Can you work these out from the drawing? Everything is in mm from the part's minimum corner. Coordinates: 2 decimals unless noted, no trailing zeros. Write each loop counter-clockwise with the first axis right and the second up, starting at its lowest first coordinate (ties: lowest second). Pieces come first, ordered by that corner, then holes.
(1) Imagine slicing it at C-C, the plane y = 450. List the corners of the cut face in (x, z) for me.
(2) For pin 1 Ø10 at (y, z) = (107.5, 7) entering from -X; pin 2 Ø12 at (y, z) = (646.5, 8.5) entering from -X, each with a flat end and sliding along its axis, tell me the tip position at first contact or that it passes through.
(3) Imagine slicing it at D-D, the plane y = 982. List the corners of the cut face in (x, z) for me.
(4) Imagine slicing it at A-A, the plane x = 766.5. List the corners of the cut face in (y, z) for me, plus the area to 3 significant figures.
(5) Imagine slicing it at B-B, the plane z = 14.5. List the corners of the cut face in (x, y) for me.
(6) Please list where these lines run through material, in increasing order: probe 1 along Y at (x, z) = (915, 17); probe 2 along X at (y, z) = (548, 7.75); probe 3 along X at (y, z) = (620, 4.5).
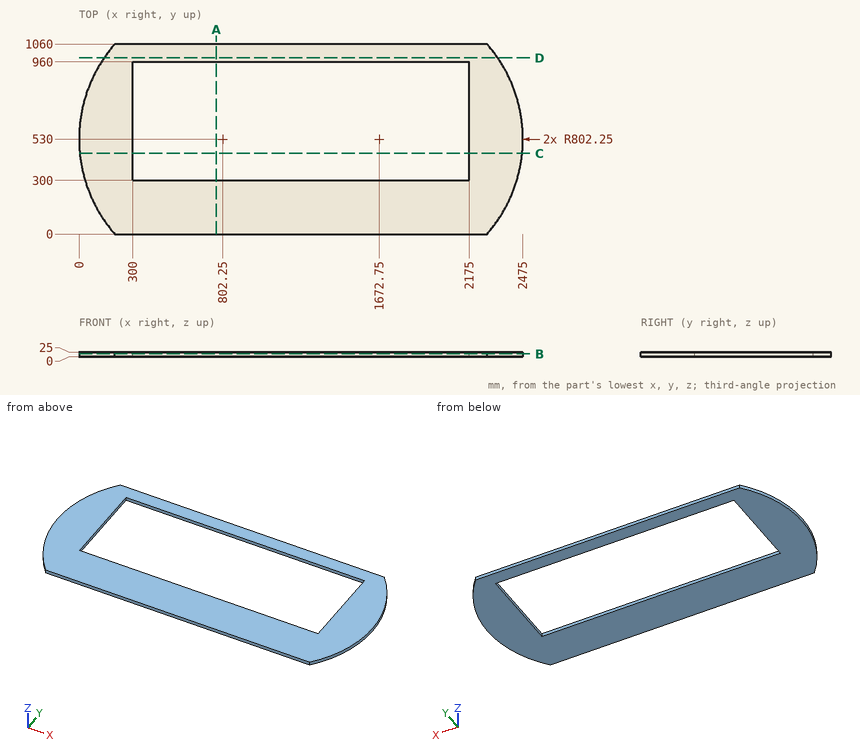
Recorded:
1. outline: (4, 0) - (300, 0) - (300, 25) - (4, 25) - close; (2175, 0) - (2471, 0) - (2471, 25) - (2175, 25) - close
2. pin 1: stops at x = 117.2
2. pin 2: stops at x = 7.65
3. outline: (139.45, 0) - (2335.55, 0) - (2335.55, 25) - (139.45, 25) - close
4. outline: (0, 0) - (300, 0) - (300, 25) - (0, 25) - close; (960, 0) - (1060, 0) - (1060, 25) - (960, 25) - close
4. area: 10,000 mm2
5. outline: (200, 0) - (2275, 0) arc R802.25 ccw to (2275, 1060) - (200, 1060) arc R802.25 ccw to start; hole (300, 300) - (2175, 300) - (2175, 960) - (300, 960) - close
6. probe 1: y = 0 to 300, 960 to 1060
6. probe 2: x = 0.2 to 300, 2175 to 2474.8
6. probe 3: x = 5.06 to 300, 2175 to 2469.94
